CAD build for the part. Positions are in the model's coordinates, mm. A direction names the side the tool comes from. Round coordinates to 2 decimals unless told otherwise and drop trailing zeros. Loops run counter-clockwise (first coordinate to the right, second up) from the corner with the lowest first, then second, coordinate; pieces in that order, holes last. Notation, with made-up numbers: M -16.5,-25 L 30.5,-25 A24 cw 30.5,-1 Z; hole C 37,-14 d2. An arc over 180 degrees is marked long. Use one line per item in the form item = value.
from build123d import *

# Parameters (mm, degrees)
BOSS_EXTRUDE1_DEPTH = 5
BOSS_EXTRUDE2_START = 8
SKETCH2_R           = 12.5
BOSS_EXTRUDE2_DEPTH = 8
CUT_EXTRUDE1_REACH  = 91.615
SKETCH3_R           = 12.5
SKETCH5_R           = 13
BOSS_EXTRUDE3_DEPTH = 12
SKETCH6_R           = 18
SKETCH6_R_2         = 13
BOSS_EXTRUDE4_DEPTH = 16
CUT_EXTRUDE2_REACH  = 160.918
SKETCH7_R           = 12.5
BOSS_EXTRUDE5_DEPTH = 12


with BuildPart() as part:
    # Sketch1 → Boss-Extrude1 (new, symmetric)
    with BuildSketch(Plane.XY):
        with BuildLine():
            Line((27.199616854, 56.153190853), (27.199616854, 72.153190853))
            Line((27.199616854, 72.153190853), (52.199616854, 72.153190853))
            Line((52.199616854, 72.153190853), (52.199616854, -7.846809147))
            Line((52.199616854, -7.846809147), (25.199616854, -23.435266415))
            ThreePointArc((25.199616854, -23.435266415), (3.94149511, -21.027797399), (0, 0))
            Line((0, 0), (27.199616854, 56.153190853))
        make_face()
    boss_extrude1 = extrude(amount=BOSS_EXTRUDE1_DEPTH, both=True)

    # Sketch2 → Boss-Extrude2 (add)
    with BuildSketch(Plane.XY.offset(5).offset(BOSS_EXTRUDE2_START)):
        with BuildLine():
            ThreePointArc((34.199616854, -7.846809147), (20.224967561, 9.697322399), (0, 0))
            ThreePointArc((0, 0), (3.94149511, -21.027797399), (25.199616854, -23.435266415))
            ThreePointArc((25.199616854, -23.435266415), (31.788074122, -16.846809147), (34.199616854, -7.846809147))
        make_face()
        with Locations((16.199616854, -7.846809147)):
            Circle(SKETCH2_R, mode=Mode.SUBTRACT)
    boss_extrude2 = extrude(amount=-BOSS_EXTRUDE2_DEPTH)

    # Sketch3 → Cut-Extrude1 (cut, up to next)
    with BuildSketch(Plane.XY.offset(5), mode=Mode.PRIVATE) as cut_extrude1_sk1:
        with Locations(Location((16.199616854, -7.846809147, 0), (0, 0, 180))):
            Circle(SKETCH3_R)
    cut_extrude1_tool1 = extrude(cut_extrude1_sk1.sketch, amount=-CUT_EXTRUDE1_REACH, mode=Mode.PRIVATE) & part.part
    add(cut_extrude1_tool1.solids().sort_by_distance((16.199617, -7.846809, 5))[0], mode=Mode.SUBTRACT)

    # Sketch5 → Boss-Extrude3 (add)
    with BuildSketch(Plane(origin=(52.199616854, 0, 0), x_dir=(0, 0, -1), z_dir=(1, 0, 0))):
        with BuildLine():
            Line((11.376048584, 121.154327694), (-5, 88.153190853))
            Line((-5, 88.153190853), (-5, 72.153190853))
            Line((-5, 72.153190853), (60, 72.153190853))
            Line((60, 72.153190853), (60, 88.153190853))
            Line((60, 88.153190853), (43.623951416, 121.154327694))
            ThreePointArc((43.623951416, 121.154327694), (27.5, 131.153190853), (11.376048584, 121.154327694))
        make_face()
        with Locations(Location((27.5, 113.153190853, 0), (0, 0, 90))):
            Circle(SKETCH5_R, mode=Mode.SUBTRACT)
    extrude(amount=-BOSS_EXTRUDE3_DEPTH)

    # Sketch6 → Boss-Extrude4 (add)
    with BuildSketch(Plane(origin=(52.199616854, 0, 0), x_dir=(0, 0, -1), z_dir=(1, 0, 0))):
        with Locations(Location((27.5, 113.153190853, 0), (0, 0, 90))):
            Circle(SKETCH6_R)
        with Locations(Location((27.5, 113.153190853, 0), (0, 0, 90))):
            Circle(SKETCH6_R_2, mode=Mode.SUBTRACT)
    extrude(amount=-BOSS_EXTRUDE4_DEPTH)

    # Mirror1: Boss-Extrude1, Boss-Extrude2 across plane
    add(boss_extrude1.mirror(Plane.XY.offset(-27.5)))
    add(boss_extrude2.mirror(Plane.XY.offset(-27.5)))

    # Sketch7 → Cut-Extrude2 (cut, up to next)
    with BuildSketch(Plane(origin=(0, 0, -60), x_dir=(-1, 0, 0), z_dir=(0, 0, -1)), mode=Mode.PRIVATE) as cut_extrude2_sk1:
        with Locations((-16.199616854, -7.846809147)):
            Circle(SKETCH7_R)
    cut_extrude2_tool1 = extrude(cut_extrude2_sk1.sketch, amount=-CUT_EXTRUDE2_REACH, mode=Mode.PRIVATE) & part.part
    add(cut_extrude2_tool1.solids().sort_by_distance((16.199617, -7.846809, -60))[0], mode=Mode.SUBTRACT)

    # Sketch8 → Boss-Extrude5 (add)
    with BuildSketch(Plane.ZY.offset(-40.199616854)):
        with BuildLine():
            Line((-5, 26.153190853), (-16.5, 26.153190853))
            Line((-16.5, 26.153190853), (-16.5, 52.153190853))
            ThreePointArc((-16.5, 52.153190853), (-27.5, 63.153190853), (-38.5, 52.153190853))
            Line((-38.5, 52.153190853), (-38.5, 26.153190853))
            Line((-38.5, 26.153190853), (-50, 26.153190853))
            Line((-50, 26.153190853), (-50, 72.153190853))
            Line((-50, 72.153190853), (-5, 72.153190853))
            Line((-5, 72.153190853), (-5, 26.153190853))
        make_face()
    extrude(amount=-BOSS_EXTRUDE5_DEPTH)


solid = part.part
1. Cut at B-B on y = -2. Write the cut outline in (x, z), and give its area (3 significant figures).
Completed:
outline = M -0.82,-68 L 5.15,-68 L 5.15,-50 L -0.82,-50 Z; M -0.82,-5 L 5.15,-5 L 5.15,13 L -0.82,13 Z; M 27.25,-68 L 33.22,-68 L 33.22,-60 L 52.2,-60 L 52.2,-50 L 27.25,-50 Z; M 27.25,-5 L 52.2,-5 L 52.2,5 L 33.22,5 L 33.22,13 L 27.25,13 Z
area = 810 mm2
2. Probe line 1 along Z through (x, y) = (37, 39); line 2 along Y through (x, z) = (8.5, 8.5); line 3 along X through (y, z) = (40, -45.5). List the from-to ranges inside material, lowest first. Write a range as from..to.
Completed:
line_1 = -60..-50, -5..5
line_2 = -24.12..-17.69, 2..8.42
line_3 = 40.2..52.2
3. Tool access for faces 4 (the face through (42.53, 131.11, -26.24)), 5 (the face through (46, 39, -38.5)), 6 (the face through (27.2, 64, 0)), 7 (the face through (32, 13, -5)): list every direction of +Z, -Z, +X, -X, +Y, -Y with a clear straight run to the whole face (end or side of a thin tool).
Completed:
face_4 = -X
face_5 = +X, -X, -Y
face_6 = +Z, -Z, -X, +Y
face_7 = -X, -Y
4. Pull direction Y, two halves, no side cores. Call faces 1 (the face through (4, -12, -68)), 2 (the face through (44.312, 100.166, -26.928)), 3 (the face through (38.89, -15.53, 0.07)): +Y half, -Y half, draft (parallel to the pull), parting line (faces both ways), or undercut.
Completed:
face_1 = draft
face_2 = undercut
face_3 = -Y half
5. Cut at D-D on z = -58. Write the cut outline in (x, y), and give its area (3 significant figures).
Completed:
outline = M 0,0 A18 ccw 25.2,-23.44 L 52.2,-7.85 L 52.2,92.18 L 40.2,92.18 L 40.2,72.15 L 27.2,72.15 L 27.2,56.15 Z; hole C 16.2,-7.85 d25
area = 3,360 mm2
6. Cut at A-A on z = -27.5. Write the cut outline in (x, y).
Completed:
outline = M 36.2,95.15 L 40.2,95.15 L 40.2,63.15 L 52.2,63.15 L 52.2,100.15 L 36.2,100.15 Z; M 36.2,126.15 L 52.2,126.15 L 52.2,131.15 L 36.2,131.15 Z
7. Drop flat-ended pins along their axis: P1, Ø5, axis at x = 42.5, z = -40.5, coming from the -Y side; P2, Ø8, axis at x = 30, y = 91, coming from the -Z side; P3, Ø11, axis at y = 65, z = -53.5, coming from the -X side; P4, Ø13, axis at x = 46.5, y = 41, coming from the +Z side. Give the stop position or say it passes through.
Completed:
P1 = 26.15
P2 = through
P3 = 27.2
P4 = 5
8. Cut at C-C on x = 44.5. Write the cut outline in (y, z).
Completed:
outline = M -12.29,-60 L 88.15,-60 L 121.15,-43.62 A18 ccw 121.15,-11.38 L 88.15,5 L -12.29,5 L -12.29,-5 L 26.15,-5 L 26.15,-16.5 L 52.15,-16.5 A11 cw 52.15,-38.5 L 26.15,-38.5 L 26.15,-50 L -12.29,-50 Z; hole C 113.15,-27.5 d26
